The listing builds one solid part. Answer for the finished solid, in the listing's coordinates (mm). Face numbers are marked on the shaded views. A direction names the side the tool comes from. Coordinates: 2 decimals unless noted, no trailing zeros. Order: outer loops, then holes, each group sorted by start corner. A loop starts at its lowest first (then second) coordinate and runs counter-clockwise, first axis right, second up. Notation, with made-up numbers: M 75.5,6.5 L 85.5,6.5 A25 cw 85.5,43.5 Z; hole C 35.25,22.25 d9. An arc over 180 degrees is marked long. One line per item, written item: value. Start each with the question number.
Q1. The part is cut by section A-A on x = 11. Give the vertices of the cut face in (y, z), then the cut area to 3 significant figures.
Q2. The part is cut by section B-B on z = 10. Give the vertices of the cut face in (x, y).
Q3. Each of these flat-tipped pins is pushed along its axis until it touches: pin 1 Ø5 at (x, y) = (11, 10) entering from +Z; pin 2 Ø8 at (y, z) = (2, 10) entering from +X. Where does it stop, or does it pass through?
Q4. The part is cut by section D-D on x = 2.25. Give the vertices of the cut face in (y, z), then the cut area to 3 significant figures.
Q5. For the marked faces 1 and 2, determine the directions among +Z, -Z, +X, -X, +Y, -Y from which every point of the face is accessible in a straight line to the end or side of a thin tool.
Q6. Determine the mould class of the marked faces 3, 4 and 5 for opening direction X: pulls with the +X half, pulls with the -X half, needs draft (parallel to the pull), parting line crosses it, or undercut.
Q7. The part is cut by section C-C on y = 9.5. Give the vertices of the cut face in (x, z).
Q8. Straight lines are drawn through the part: line 1 along Y through (x, z) = (2.3, 10); line 2 along Y through (x, z) = (11, 2.8); line 3 along Z through (x, y) = (10, 3.25). For each, find the intervals that lie inside material, in ascending order. Write a range as [from, to].
```python
from build123d import *

# Parameters (mm, degrees)
BOSS_EXTRUDE1_DEPTH = 15
SKETCH2_R           = 2
CUT_EXTRUDE1_DEPTH  = 25.103941586
SKETCH3_R           = 1.25
CUT_EXTRUDE2_DEPTH  = 27.570660511


with BuildPart() as part:
    # Sketch1 → Boss-Extrude1 (new, symmetric)
    with BuildSketch(Plane(origin=(0, 0, 0), x_dir=(1, 0, 0), z_dir=(0, 1, 0))):
        Polygon((0, 0), (16, 0), (16, -5), (5, -5), (5, -15), (0, -15), align=None)
    extrude(amount=BOSS_EXTRUDE1_DEPTH, both=True)

    # Sketch2 → Cut-Extrude1 (cut, through all)
    with BuildSketch(Plane.XY.offset(5)):
        with Locations((11, 10)):
            Circle(SKETCH2_R)
        with Locations((11, -10)):
            Circle(SKETCH2_R)
    extrude(amount=-CUT_EXTRUDE1_DEPTH, mode=Mode.SUBTRACT)

    # Sketch3 → Cut-Extrude2 (cut, through all)
    with BuildSketch(Plane.ZY):
        with Locations((10, 9.5)):
            Circle(SKETCH3_R)
        with Locations((10, -9.5)):
            Circle(SKETCH3_R)
    extrude(amount=-CUT_EXTRUDE2_DEPTH, mode=Mode.SUBTRACT)


solid = part.part
```
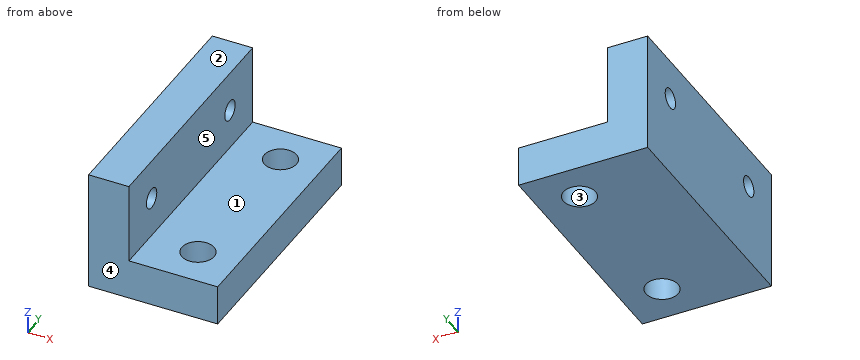
Output:
1. outline: M -15,0 L -12,0 L -12,5 L -15,5 Z; M -8,0 L 8,0 L 8,5 L -8,5 Z; M 12,0 L 15,0 L 15,5 L 12,5 Z
1. area: 110 mm^2
2. outline: M 0,-15 L 5,-15 L 5,-10.75 L 0,-10.75 Z; M 0,-8.25 L 5,-8.25 L 5,8.25 L 0,8.25 Z; M 0,10.75 L 5,10.75 L 5,15 L 0,15 Z
3. pin 1: stops at z = 5
3. pin 2: stops at x = 5
4. outline: M -15,0 L 15,0 L 15,15 L -15,15 Z; hole C -9.5,10 d2.5; hole C 9.5,10 d2.5
4. area: 440 mm^2
5. face 1: +Z, +X, +Y, -Y
5. face 2: +Z, +X, -X, +Y, -Y
6. face 3: undercut
6. face 4: needs draft
6. face 5: pulls with the +X half
7. outline: M 0,0 L 9.06,0 L 9.06,5 L 5,5 L 5,8.75 L 0,8.75 Z; M 0,11.25 L 5,11.25 L 5,15 L 0,15 Z; M 12.94,0 L 16,0 L 16,5 L 12.94,5 Z
8. line 1: y = [-15, -10.75], [-8.25, 8.25], [10.75, 15]
8. line 2: y = [-15, -12], [-8, 8], [12, 15]
8. line 3: z = [0, 5]
